Check sheet for the modelled part. Datum: model origin and axes. Units: mm. A direction names the side the tool comes from. Give positions to 0.01 mm unless a question says otherwise; leave off trailing zeros. Order: outer loops, then holes, each group sorted by start corner. A loop starts at its lowest first (then second) coordinate and runs counter-clockwise, first axis right, second up. Notation, with made-up numbers: (14.25, -26.5) -> (18.25, -26.5) arc R12 ccw to (18.25, -11.5) -> close; hole circle Ø5 at (-38, 53). An arc over 180 degrees is marked (long way). Answer in a Markdown table with one row per item. Add a question column.
(1) Set-up check for faces 4 (the face through (-800.66, -621.59, 2377.13)), 5 (the face through (-665.514, -360, 1825)), 6 (the face through (-995.514, -360, 1824)): record each of +Z, -Z, +X, -X, +Y, -Y from which the full face is reachable in a straight line by a thin tool's end or side.
(2) Cross-section at A-A (x = -954). Record the cut outline in (y, z), then the cut area to 3 significant figures.
(3) Release check for a two-part mould opening along Y. For faces 1 (the face through (-850.89, -461.25, 2129.35)), 2 (the face through (-803.921, -626.484, 2385.911)), 3 (the face through (-730.404, -371.062, 1853.455)) record: released by +Y, released by -Y, zero draft, split by the parting line, or undercut.
(4) Thickness scan on L1, parallel to X at y = -465, z = 2109; L2, parallel to X at y = -634, z = 2202.5; L3, parallel to Z at x = -762.5, y = -334.5. Record the ranges inside material, lowest first. Write a range as [from, to].
(5) Go/stop test with flat-tipped pins: pin 1 (2 mm diameter, centred on y = -452, z = 2224.5, fed in from +X); pin 2 (3 mm diameter, centred on y = -470, z = 1955.5, fed in from +X); pin 3 (3.5 mm diameter, centred on x = -714.5, z = 1831.5, fed in from -Y). Record where each tip stops, or that it passes through.
```python
from build123d import *

# Parameters (mm, degrees)
CROQUIS2_R              = 25.000000002
SALIENTE_EXTRUIR1_DEPTH = 200
SALIENTE_EXTRUIR3_START = -550
CROQUIS5_R              = 125
CROQUIS5_R_2            = 110
SALIENTE_EXTRUIR3_DEPTH = 600
CROQUIS6_R              = 125
CROQUIS6_R_2            = 75
SALIENTE_EXTRUIR4_DEPTH = 10
REDONDEO1_R             = 10
SALIENTE_EXTRUIR5_START = -10
CROQUIS7_R              = 125
SALIENTE_EXTRUIR5_DEPTH = 10
SALIENTE_EXTRUIR7_DEPTH = 130


with BuildPart() as part:
    # Croquis2 → Saliente-Extruir1 (new body)
    with BuildSketch(Plane.ZY.offset(995.514439922)):
        with Locations((1824.824247225, -360.492761656)):
            Circle(CROQUIS2_R)
    extrude(amount=-SALIENTE_EXTRUIR1_DEPTH)

    # Croquis5 → Saliente-Extruir3 (add)
    with BuildSketch(Plane(origin=(0, -1175.698746169, 2749.222800852), x_dir=(1, 0, 0), z_dir=(0, -0.39320162856731994, 0.919452271350725)).offset(SALIENTE_EXTRUIR3_START)):
        with Locations(Location((-728.864439922, 386.067977351, 0), (0, 0, 270))):
            Circle(CROQUIS5_R)
        with Locations(Location((-728.864439922, 386.067977351, 0), (0, 0, 270))):
            Circle(CROQUIS5_R_2, mode=Mode.SUBTRACT)
    extrude(amount=-SALIENTE_EXTRUIR3_DEPTH)

    # Croquis6 → Saliente-Extruir4 (add)
    with BuildSketch(Plane(origin=(0, -959.437850457, 2243.524051609), x_dir=(1, 0, 0), z_dir=(0, -0.39320162856732, 0.919452271350725))):
        with Locations(Location((-728.864439922, 386.067977351, 0), (0, 0, 270))):
            Circle(CROQUIS6_R)
        with Locations(Location((-728.864439922, 386.067977351, 0), (0, 0, 270))):
            Circle(CROQUIS6_R_2, mode=Mode.SUBTRACT)
    extrude(amount=-SALIENTE_EXTRUIR4_DEPTH)

    # Redondeo1
    redondeo1_edges = [part.edges().sort_by_distance(p)[0] for p in [
        (-728.864439922, -489.535237867, 2444.476812612),
    ]]
    fillet(redondeo1_edges, radius=REDONDEO1_R)

    # Croquis7 → Saliente-Extruir5 (add)
    with BuildSketch(Plane(origin=(0, -723.516873317, 1691.852688798), x_dir=(-1, 0, 0), z_dir=(0, 0.39320162856732, -0.919452271350725)).offset(SALIENTE_EXTRUIR5_START)):
        with Locations(Location((728.864439922, 386.067977351, 0), (0, 0, 270))):
            Circle(CROQUIS7_R)
    extrude(amount=SALIENTE_EXTRUIR5_DEPTH)

    # Croquis11 → Saliente-Extruir7 (add)
    with BuildSketch(Plane(origin=(-795.514439922, 0, 0), x_dir=(0, 0, -1), z_dir=(1, 0, 0))):
        with BuildLine():
            Line((-1850.902577314, -351.598827639), (-1842.90075375, -343.22313769))
            ThreePointArc((-1842.90075375, -343.22313769), (-1801.83794044, -350.662720941), (-1824.824247225, -385.492761657))
            Line((-1824.824247225, -385.492761657), (-1836.407915144, -385.492761657))
            Line((-1836.407915144, -385.492761657), (-1850.902577314, -351.598827639))
        make_face()
    extrude(amount=SALIENTE_EXTRUIR7_DEPTH)


solid = part.part
```
Answer below:
| question | item | result |
|---|---|---|
| 1 | face 4 | none |
| 1 | face 5 | -Z, +X, +Y |
| 1 | face 6 | +Z, -Z, -X, +Y, -Y |
| 2 | outline | circle Ø50 at (-360.49, 1824.82) |
| 2 | area | 1,960 mm² |
| 3 | face 1 | split by the parting line |
| 3 | face 2 | released by -Y |
| 3 | face 3 | undercut |
| 4 | L1 | x = [-852.88, -837.75], [-619.98, -604.85] |
| 4 | L2 | x = [-799.73, -767.55], [-690.18, -658] |
| 4 | L3 | z = [1858.21, 1869.09], [2030.4, 2070.22] |
| 5 | pin 1 | stops at x = -626.69 |
| 5 | pin 2 | stops at x = -613.37 |
| 5 | pin 3 | stops at y = -499.18 |
